Check sheet for the modelled part. Datum: model origin and axes. Units: mm. A direction names the side the tool comes from. Coordinates: 2 decimals unless noted, no trailing zeros. Write each loop counter-clockwise with the first axis right and the second up, starting at its lowest first coordinate (ties: lowest second). Pieces come first, ordered by that corner, then holes. Notation, with made-up numbers: M 51.25,62 L 72.25,62 A27 cw 72.25,88 Z; hole C 79,51 d3. An arc over 180 degrees is marked long. Answer as CSV lines item,"result". Start each with the question number.
1) Access from +Z, -Z, +X, -X, +Y, -Y to the whole of each face (thin tool, end or side, straight path). Record for faces 1 (the flat face through (-12, -3, 2)), 2 (the flat face through (12, -3, 2)), 3 (the flat face through (-12, 3, 2)), 4 (the flat face through (5, -1, 1.5)), 5 (the cylindrical face through (0, -11, 2)).
2) Draft check along Y on faces 6 (the flat face through (-2, 5, 1.5)), 7 (the flat face through (12, 3, 2)), 8 (the cylindrical face through (-16, 0, 2)). Enter one of: +Y half, -Y half, draft (parallel to the pull), parting line (faces both ways), or undercut.
3) Section check B-B (x = -1.5). Record the cut outline in (y, z), and give its area (3 significant figures).
4) Go/stop test with flat-tipped pins: pin 1 Ø2.5 at (x, y) = (4.25, 0) entering from +Z; pin 2 Ø1.9 at (x, z) = (12, 1.5) entering from +Y; pin 3 Ø1.5 at (y, z) = (6, 3.5) entering from +X; pin 4 Ø1.2 at (x, y) = (-2.13, -3.68) entering from -Z (3 decimals). Record where each tip stops, or that it passes through.
5) Section check D-D (x = 4). Record the cut outline in (y, z), and give its area (3 significant figures).
6) Section check C-C (z = 0.85). Record the cut outline in (x, y) (3 decimals), and give its area (3 significant figures).
7) Material ranges on L1, parallel to X at y = 0, z = 1.2; L2, parallel to X at y = 0.75, z = 0.65; L3, parallel to Y at x = -2, z = 0.8, recorded low to high. Write a range as [from, to].
8) Section check A-A (y = 0). Record the cut outline in (x, z).
from build123d import *

# Parameters (mm, degrees)
CYLINDER150_R     = 1.7
CYLINDER150_DEPTH = 11
CYLINDER151_R     = 1.7
CYLINDER151_DEPTH = 11
CYLINDER157_R     = 2.25
CYLINDER157_DEPTH = 8
CYLINDER156_R     = 1
CYLINDER156_DEPTH = 5
CYLINDER147_R     = 1
CYLINDER147_DEPTH = 1
ARRAY_COUNT       = 3
BOX_W             = 3
BOX_H             = 6
BOX_DEPTH         = 4
CYLINDER153_R     = 11
CYLINDER153_DEPTH = 4
BOX001_W          = 3
BOX001_H          = 6
BOX001_DEPTH      = 4
CYLINDER158_R     = 3
CYLINDER158_DEPTH = 4
CYLINDER_R        = 3
CYLINDER_DEPTH    = 4


with BuildPart() as obj1:
    # Cylinder150 → Cylinder150 (new body)
    with BuildSketch(Plane(origin=(-13, 0, 0), x_dir=(1, 0, 0), z_dir=(0, 0, 1))):
        Circle(CYLINDER150_R)
    extrude(amount=CYLINDER150_DEPTH)


with BuildPart() as obj2:
    # Cylinder151 → Cylinder151 (new body)
    with BuildSketch(Plane(origin=(13, 0, 0), x_dir=(1, 0, 0), z_dir=(0, 0, 1))):
        Circle(CYLINDER151_R)
    extrude(amount=CYLINDER151_DEPTH)


with BuildPart() as sealsubtraction:
    # Cylinder157 → Cylinder157 (new body)
    with BuildSketch(Plane.XY.offset(1.5)):
        Circle(CYLINDER157_R)
    extrude(amount=CYLINDER157_DEPTH)


with BuildPart() as bottomwireoutlet:
    # Cylinder156 → Cylinder156 (new body)
    with BuildSketch(Plane.XY.offset(-2)):
        Circle(CYLINDER156_R)
    extrude(amount=CYLINDER156_DEPTH)


with BuildPart() as fusion013:
    # Cylinder147 → Cylinder147 (new body)
    with BuildSketch(Plane.XY.offset(4.5)):
        Circle(CYLINDER147_R)
    extrude(amount=CYLINDER147_DEPTH)

    # Fusion: union SealSubtraction, BottomWireOutlet
    add(sealsubtraction.part)
    add(bottomwireoutlet.part)


with BuildPart() as fusion013_1:
    # Fusion placement: moved
    add(fusion013.part.moved(Location((4.25, 0, 0))))

    # Array: Fusion013 ×3 about axis
    array_axis = Axis((0, 0, 0), (0, 0, 1))


with BuildPart() as fusion013_2:
    add(fusion013_1.part)
    for i in range(1, ARRAY_COUNT):
        add(fusion013_1.part.rotate(array_axis, i * 360 / ARRAY_COUNT))

    # Fusion013: union obj1, obj2
    add(obj1.part)
    add(obj2.part)


with BuildPart() as mountcube1:
    # Box → Box (new body)
    with BuildSketch(Plane(origin=(-13, -3, 0), x_dir=(1, 0, 0), z_dir=(0, 0, 1))):
        with Locations((1.5, 3)):
            Rectangle(BOX_W, BOX_H)
    extrude(amount=BOX_DEPTH)


with BuildPart() as body:
    # Cylinder153 → Cylinder153 (new body)
    with BuildSketch(Plane.XY):
        Circle(CYLINDER153_R)
    extrude(amount=CYLINDER153_DEPTH)


with BuildPart() as mountcube002:
    # Box001 → Box001 (new body)
    with BuildSketch(Plane(origin=(10, -3, 0), x_dir=(1, 0, 0), z_dir=(0, 0, 1))):
        with Locations((1.5, 3)):
            Rectangle(BOX001_W, BOX001_H)
    extrude(amount=BOX001_DEPTH)


with BuildPart() as mountflange002:
    # Cylinder158 → Cylinder158 (new body)
    with BuildSketch(Plane(origin=(13, 0, 0), x_dir=(1, 0, 0), z_dir=(0, 0, 1))):
        Circle(CYLINDER158_R)
    extrude(amount=CYLINDER158_DEPTH)


with BuildPart() as cut:
    # Cylinder → Cylinder (new body)
    with BuildSketch(Plane(origin=(-13, 0, 0), x_dir=(1, 0, 0), z_dir=(0, 0, 1))):
        Circle(CYLINDER_R)
    extrude(amount=CYLINDER_DEPTH)

    # Fusion012: union MountCube1, Body, MountCube002, MountFlange002
    add(mountcube1.part)
    add(body.part)
    add(mountcube002.part)
    add(mountflange002.part)

    # Cut: cut Fusion013
    add(fusion013_2.part, mode=Mode.SUBTRACT)


solid = cut.part
Results found:
1,face 1,"+Z, -Z, -X, -Y"
1,face 2,"+Z, -Z, +X, -Y"
1,face 3,"+Z, -Z, -X, +Y"
1,face 4,"+Z"
1,face 5,"+Z, -Z, -Y"
2,face 6,"undercut"
2,face 7,"+Y half"
2,face 8,"parting line"
3,outline,"M -10.9,0 L -4.46,0 L -4.46,1.5 L -5.84,1.5 L -5.84,4 L -10.9,4 Z; M -2.9,0 L 2.9,0 L 2.9,1.5 L 1.52,1.5 L 1.52,4 L -1.52,4 L -1.52,1.5 L -2.9,1.5 Z; M 4.46,0 L 10.9,0 L 10.9,4 L 5.84,4 L 5.84,1.5 L 4.46,1.5 Z"
3,area,"60.9 mm2"
4,pin 1,"stops at z = 1.5"
4,pin 2,"stops at y = 3"
4,pin 3,"stops at x = 9.67"
4,pin 4,"passes through"
5,outline,"M -10.25,0 L -0.97,0 L -0.97,1.5 L -2.24,1.5 L -2.24,4 L -10.25,4 Z; M 0.97,0 L 10.25,0 L 10.25,4 L 2.24,4 L 2.24,1.5 L 0.97,1.5 Z"
5,area,"67.9 mm2"
6,outline,"M -13,-3 L -10.583,-3 A11 ccw 10.583,-3 L 13,-3 A3 ccw 13,3 L 10.583,3 A11 ccw -10.583,3 L -13,3 A3 ccw Z; hole C -13,0 d3.4; hole C -2.125,-3.681 d2; hole C -2.125,3.681 d2; hole C 4.25,0 d2; hole C 13,0 d3.4"
6,area,"406 mm2"
7,L1,"x = [-16, -14.7], [-11.3, 3.25], [5.25, 11.3], [14.7, 16]"
7,L2,"x = [-15.9, -14.53], [-11.47, 3.59], [4.91, 11.47], [14.53, 15.9]"
7,L3,"y = [-10.82, -4.67], [-2.69, 2.69], [4.67, 10.82]"
8,outline,"M -16,0 L -14.7,0 L -14.7,4 L -16,4 Z; M -11.3,0 L 3.25,0 L 3.25,1.5 L 2,1.5 L 2,4 L -11.3,4 Z; M 5.25,0 L 11.3,0 L 11.3,4 L 6.5,4 L 6.5,1.5 L 5.25,1.5 Z; M 14.7,0 L 16,0 L 16,4 L 14.7,4 Z"
